Source: CAD feature listing. Evaluate the final solid. Frame: model axes, mm. A direction names the side the tool comes from. Coordinates: 2 decimals unless noted, no trailing zeros. Write each loop counter-clockwise with the first axis right and the second up, starting at its lowest first coordinate (ties: lowest second). Pieces come first, ordered by that corner, then holes. Notation, with made-up numbers: (-1.5, 79.5) -> (10.5, 79.5) arc R20 cw to (10.5, 105.5) -> close; hole circle Ø8 at (-23.75, 69.25). An arc over 180 degrees is marked (long way). Write item = value, one per line.
from build123d import *

# Parameters (mm, degrees)
SKETCH1_R           = 1.75
BOSS_EXTRUDE1_DEPTH = 8.5
FILLET1_R           = 3
SKETCH3_R           = 4.25
CUT_EXTRUDE3_DEPTH  = 5
CUT_EXTRUDE4_REACH  = 50.428
BOSS_EXTRUDE2_DEPTH = 4
CUT_EXTRUDE5_REACH  = 81.418


with BuildPart() as part:
    # Sketch1 → Boss-Extrude1 (new, symmetric)
    with BuildSketch(Plane(origin=(0, 0, 0), x_dir=(0, 0, -1), z_dir=(1, 0, 0))):
        with BuildLine():
            ThreePointArc((0, 3), (-2.121320344, 2.121320344), (-3, 0))
            Line((-3, 0), (-3, -5))
            Line((-3, -5), (1.279790789, -5))
            Line((1.279790789, -5), (47, -1))
            Line((47, -1), (47, 3))
            Line((47, 3), (0, 3))
        make_face()
        Circle(SKETCH1_R, mode=Mode.SUBTRACT)
    extrude(amount=BOSS_EXTRUDE1_DEPTH, both=True)

    # Fillet1
    fillet1_edges = [part.edges().sort_by_distance(p)[0] for p in [
        (0, -5, 3),
    ]]
    fillet(fillet1_edges, radius=FILLET1_R)

    # Sketch3 → Cut-Extrude3 (cut)
    with BuildSketch(Plane(origin=(0, 3, 0), x_dir=(1, 0, 0), z_dir=(0, 1, 0))):
        with Locations(Location((0, 27, 0), (0, 0, 270))):
            Circle(SKETCH3_R)
    extrude(amount=-CUT_EXTRUDE3_DEPTH, mode=Mode.SUBTRACT)

    # Sketch4 → Cut-Extrude4 (cut, up to next)
    with BuildSketch(Plane(origin=(0, 3, 0), x_dir=(1, 0, 0), z_dir=(0, 1, 0)), mode=Mode.PRIVATE) as cut_extrude4_sk1:
        with BuildLine():
            Line((-8.5, -3), (-5, -3))
            Line((-5, -3), (-5, 32.6))
            ThreePointArc((-5, 32.6), (-5.995836944, 35.004163056), (-8.4, 36))
            Line((-8.4, 36), (-8.5, 36))
            Line((-8.5, 36), (-8.5, -3))
        make_face()
    cut_extrude4_tool1 = extrude(cut_extrude4_sk1.sketch, amount=-CUT_EXTRUDE4_REACH, mode=Mode.PRIVATE) & part.part
    # Sketch4 → Cut-Extrude4 (cut, up to next)
    with BuildSketch(Plane(origin=(0, 3, 0), x_dir=(1, 0, 0), z_dir=(0, 1, 0)), mode=Mode.PRIVATE) as cut_extrude4_sk2:
        with BuildLine():
            Line((8.4, 36), (8.5, 36))
            Line((8.5, 36), (8.5, -3))
            Line((8.5, -3), (5, -3))
            Line((5, -3), (5, 32.6))
            ThreePointArc((5, 32.6), (5.995836944, 35.004163056), (8.4, 36))
        make_face()
    cut_extrude4_tool2 = extrude(cut_extrude4_sk2.sketch, amount=-CUT_EXTRUDE4_REACH, mode=Mode.PRIVATE) & part.part
    add(cut_extrude4_tool1.solids().sort_by_distance((-6.768336, 3, -16.153098))[0], mode=Mode.SUBTRACT)
    add(cut_extrude4_tool2.solids().sort_by_distance((6.768336, 3, -16.153098))[0], mode=Mode.SUBTRACT)

    # Sketch5 → Boss-Extrude2 (add)
    with BuildSketch(Plane(origin=(0, 3, 0), x_dir=(1, 0, 0), z_dir=(0, 1, 0))):
        with BuildLine():
            ThreePointArc((-11, 47), (-12.767766953, 47.732233047), (-13.5, 49.5))
            Line((-13.5, 49.5), (-13.5, 55.23782662))
            ThreePointArc((-13.5, 55.23782662), (-13.12012024, 56.562624781), (-12.095927867, 57.484811736))
            Line((-12.095927867, 57.484811736), (10.994949478, 68.746985116))
            ThreePointArc((10.994949478, 68.746985116), (11.528499709, 68.935925162), (12.090877345, 69))
            Line((12.090877345, 69), (25.464466094, 69))
            ThreePointArc((25.464466094, 69), (26.421174675, 68.809698831), (27.232233047, 68.267766953))
            Line((27.232233047, 68.267766953), (37.767766953, 57.732233047))
            ThreePointArc((37.767766953, 57.732233047), (38.309698831, 56.921174675), (38.5, 55.964466094))
            Line((38.5, 55.964466094), (38.5, 49.5))
            ThreePointArc((38.5, 49.5), (37.767766953, 47.732233047), (36, 47))
            Line((36, 47), (8.5, 47))
            Line((8.5, 47), (-8.5, 47))
            Line((-8.5, 47), (-11, 47))
        make_face()
        with BuildLine():
            Line((10.5, 47), (8.5, 47))
            Line((8.5, 47), (8.5, 45))
            ThreePointArc((8.5, 45), (9.085786438, 46.414213562), (10.5, 47))
        make_face()
        with BuildLine():
            Line((-8.5, 45), (-8.5, 47))
            Line((-8.5, 47), (-10.5, 47))
            ThreePointArc((-10.5, 47), (-9.085786438, 46.414213562), (-8.5, 45))
        make_face()
    extrude(amount=-BOSS_EXTRUDE2_DEPTH)

    # Sketch6 → Cut-Extrude5 (cut, up to next)
    with BuildSketch(Plane(origin=(0, 3, 0), x_dir=(1, 0, 0), z_dir=(0, 1, 0)), mode=Mode.PRIVATE) as cut_extrude5_sk1:
        with BuildLine():
            Line((5, 32.6), (5, 41.5))
            ThreePointArc((5, 41.5), (6.610912703, 45.389087297), (10.5, 47))
            Line((10.5, 47), (10.5, 32.6))
            Line((10.5, 32.6), (5, 32.6))
        make_face()
    cut_extrude5_tool1 = extrude(cut_extrude5_sk1.sketch, amount=-CUT_EXTRUDE5_REACH, mode=Mode.PRIVATE) & part.part
    # Sketch6 → Cut-Extrude5 (cut, up to next)
    with BuildSketch(Plane(origin=(0, 3, 0), x_dir=(1, 0, 0), z_dir=(0, 1, 0)), mode=Mode.PRIVATE) as cut_extrude5_sk2:
        with BuildLine():
            Line((-5, 32.6), (-10.5, 32.6))
            Line((-10.5, 32.6), (-10.5, 47))
            ThreePointArc((-10.5, 47), (-6.610912703, 45.389087297), (-5, 41.5))
            Line((-5, 41.5), (-5, 32.6))
        make_face()
    cut_extrude5_tool2 = extrude(cut_extrude5_sk2.sketch, amount=-CUT_EXTRUDE5_REACH, mode=Mode.PRIVATE) & part.part
    add(cut_extrude5_tool1.solids().sort_by_distance((7.885844, 3, -39.266841))[0], mode=Mode.SUBTRACT)
    add(cut_extrude5_tool2.solids().sort_by_distance((-7.885844, 3, -39.266841))[0], mode=Mode.SUBTRACT)


solid = part.part
1) Pull-direction query (Z, two-part tool) for faces 1 (the flat face through (0, -2, -27)), 2 (the cylindrical face through (38, 1, -48)), 3 (the flat face through (13, -1, -55)); classes: +Z half, -Z half, draft (parallel to the pull), parting line (faces both ways), or undercut.
Answer block:
face_1 = undercut
face_2 = +Z half
face_3 = draft
2) Cut plane C-C, the plane z = -27. Output: boundary loops of the cut face in (x, y), and give its area (3 significant figures).
Answer block:
outline = (-5, -2.75) -> (5, -2.75) -> (5, 3) -> (4.25, 3) -> (4.25, -2) -> (-4.25, -2) -> (-4.25, 3) -> (-5, 3) -> close
area = 15.0 mm2
3) Cut plane A-A, the plane y = 1. Output: boundary loops of the cut face in (x, z), and give its area (3 significant figures).
Answer block:
outline = (-13.5, -55.24) arc R2.5 ccw to (-12.1, -57.48) -> (10.99, -68.75) arc R2.5 ccw to (12.09, -69) -> (25.46, -69) arc R2.5 ccw to (27.23, -68.27) -> (37.77, -57.73) arc R2.5 ccw to (38.5, -55.96) -> (38.5, -49.5) arc R2.5 ccw to (36, -47) -> (10.5, -47) arc R5.5 cw to (5, -41.5) -> (5, -1.44) -> (-5, -1.44) -> (-5, -41.5) arc R5.5 cw to (-10.5, -47) -> (-11, -47) arc R2.5 ccw to (-13.5, -49.5) -> close; (-5, 1.44) -> (5, 1.44) -> (5, 2.83) -> (-5, 2.83) -> close; hole circle Ø8.5 at (0, -27)
area = 1,340 mm2
4) Cut plane B-B, the plane x = 0. Output: boundary loops of the cut face in (y, z), and give its area (3 significant figures).
Answer block:
outline = (-5, -1.28) -> (-1, -47) -> (-1, -63.38) -> (3, -63.38) -> (3, -31.25) -> (-2, -31.25) -> (-2, -22.75) -> (3, -22.75) -> (3, 0) arc R3 ccw to (0, 3) -> (-2, 3) arc R3 ccw to (-5, 0) -> close; hole circle Ø3.5 at (0, 0)
area = 318 mm2
5) Reachability of faces 4 (the flat face through (5, 0, -19)), 5 (the cylindrical face through (0.07, -4.14, 2.1)), 6 (the flat face through (-5, 0, -20)) from +Z, -Z, +X, -X, +Y, -Y: full face, straight path, thin tool, end or side. Return the list, or none.
Answer block:
face_4 = +Z, +X, +Y, -Y
face_5 = +Z, +X, -X, -Y
face_6 = +Z, -X, +Y, -Y
6) Material intervals for probe 1 along Z at (x, y) = (-1.5, -0.75); probe 2 along X at (y, z) = (0.2, -27); probe 3 along Z at (x, y) = (16.5, 1.25), sorted ascending. Write a range as [from, to].
Answer block:
probe_1 = [-62.65, -30.98], [-23.02, -1.58], [1.58, 3]
probe_2 = [-5, -4.25], [4.25, 5]
probe_3 = [-69, -47]
7) Cut plane D-D, the plane x = 24. Output: boundary loops of the cut face in (y, z).
Answer block:
outline = (-1, -69) -> (3, -69) -> (3, -47) -> (-1, -47) -> close
8) First-contact query: pin 1 Ø2.5 at (y, z) = (0.5, -26) entering from +X; pin 2 Ø5 at (x, z) = (-5.5, -42) entering from -Y; pin 3 Ø7 at (x, z) = (0, -27) entering from -Y; pin 4 Ø12 at (x, z) = (26, -45.5) entering from +Y. Flat tips, straight axial feed; report the tip coordinate or a pass-through.
Answer block:
pin_1 = 5
pin_2 = -1.65
pin_3 = -3.06
pin_4 = 3
